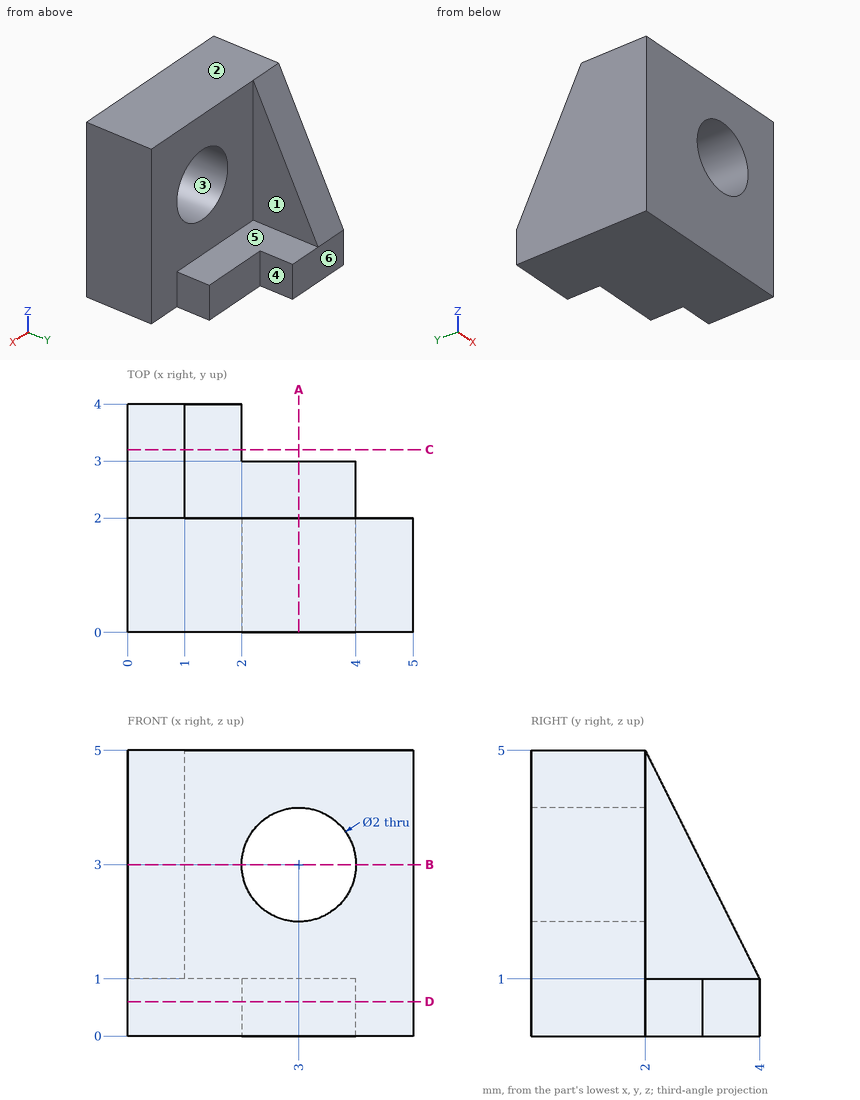
Design review of the part shown in the three views and the two pictorial views. Dimensions are in mm from the part's minimum x, y and z. A direction names the side the tool comes from. Give positions to 0.01 mm unless a question says otherwise; leave off trailing zeros. Loops run counter-clockwise (first coordinate to the right, second up) from the corner with the lowest first, then second, coordinate; pieces in that order, holes last. Notation, with made-up numbers: (5.25, 8) - (60.25, 8) arc R8 cw to (60.25, 19) - close; hole circle Ø8 at (53.5, 31). An arc over 180 degrees is marked (long way). Answer as a JSON object with one key per item and string values.
Q1. To check wall thickness, follow line 1 along Z through (x, y) = (3, 0.45); line 2 along Y through (x, z) = (1.1, 3.2). State the ranges of each line that lie inside material, in increasing order.
Worked out:
{"line 1": "z = 0 to 2, 4 to 5", "line 2": "y = 0 to 2"}
Q2. Mouldability with a two-part tool opening along Z and no side actions: class the marked faces 1, 2 and 3 as +Z half, -Z half, draft (parallel to the pull), parting line (faces both ways), or undercut.
Worked out:
{"face 1": "draft", "face 2": "+Z half", "face 3": "undercut"}
Q3. Add section D-D on z = 0.6. State the section outline as (x, y) points.
Worked out:
{"outline": "(0, 0) - (5, 0) - (5, 2) - (4, 2) - (4, 3) - (2, 3) - (2, 4) - (0, 4) - close"}
Q4. Add section A-A on x = 3. State the section outline as (y, z) points.
Worked out:
{"outline": "(0, 0) - (3, 0) - (3, 1) - (2, 1) - (2, 2) - (0, 2) - close; (0, 4) - (2, 4) - (2, 5) - (0, 5) - close"}
Q5. Add section B-B on z = 3. State the section outline as (x, y) points.
Worked out:
{"outline": "(0, 0) - (2, 0) - (2, 2) - (1, 2) - (1, 3) - (0, 3) - close; (4, 0) - (5, 0) - (5, 2) - (4, 2) - close"}
Q6. For the marked faces 4, 5 and 6, list the 3-axis set-ups (+Z, -Z, +X, -X, +Y, -Y) from which the entire face can be reached by the end or side of a thin tool; tool diameter is ignored.
Worked out:
{"face 4": "+Z, -Z, +X, +Y", "face 5": "+Z, +X, +Y", "face 6": "+Z, -Z, +X, -X, +Y"}
Q7. Insertion check: pin 1 (2 mm diameter, centred on x = 3, z = 3.5, fed in from +Y); pin 2 (1.6 mm diameter, centred on y = 3, z = 2.5, fed in from +X); pin 3 (1.8 mm diameter, centred on x = 3, z = 3, fed in from +Y). Each pin has a flat end and moves straight along its axis. Give the tip position at first contact, or say it passes through.
Worked out:
{"pin 1": "stops at y = 2", "pin 2": "stops at x = 1", "pin 3": "passes through"}
Q8. Add section C-C on y = 3.2. State the section outline as (x, z) points, plus the area to 3 significant figures.
Worked out:
{"outline": "(0, 0) - (2, 0) - (2, 1) - (1, 1) - (1, 2.6) - (0, 2.6) - close", "area": "3.60 mm^2"}
